from build123d import *

# Parameters (mm, degrees)
SKETCH1_R               = 4.60375
BOSS_EXTRUDE1_DEPTH     = 2.54
SKETCH2_R               = 3.175
BOSS_EXTRUDE2_DEPTH     = 45.72
SKETCH3_R               = 1.27
CUT_EXTRUDE1_DEPTH      = 5.60375
CUT_EXTRUDE1_DEPTH_BACK = 5.60375
FILLET1_R               = 0.635
CHAMFER1_SIZE           = 0.635
SKETCH4_W               = 16.845680721
SKETCH4_H               = 19.604839444
CUT_EXTRUDE2_DEPTH      = 5.60375
CUT_EXTRUDE2_DEPTH_BACK = 5.6037501


with BuildPart() as part:
    # Sketch1 → Boss-Extrude1 (new body)
    with BuildSketch(Plane(origin=(0, 0, 0), x_dir=(1, 0, 0), z_dir=(0, 1, 0))):
        Circle(SKETCH1_R)
    extrude(amount=BOSS_EXTRUDE1_DEPTH)

    # Sketch2 → Boss-Extrude2 (add)
    with BuildSketch(Plane(origin=(0, 2.54, 0), x_dir=(1, 0, 0), z_dir=(0, 1, 0))):
        Circle(SKETCH2_R)
    extrude(amount=BOSS_EXTRUDE2_DEPTH)

    # Sketch3 → Cut-Extrude1 (cut, two sides)
    with BuildSketch(Plane.XY) as cut_extrude1_sk:
        with Locations((0, 18.415)):
            Circle(SKETCH3_R)
        with Locations((0, 23.495)):
            Circle(SKETCH3_R)
        with Locations((0, 28.575)):
            Circle(SKETCH3_R)
        with Locations((0, 33.655)):
            Circle(SKETCH3_R)
        with Locations((0, 38.735)):
            Circle(SKETCH3_R)
        with Locations((0, 43.815)):
            Circle(SKETCH3_R)
    extrude(amount=CUT_EXTRUDE1_DEPTH, mode=Mode.SUBTRACT)
    extrude(cut_extrude1_sk.sketch, amount=-CUT_EXTRUDE1_DEPTH_BACK, mode=Mode.SUBTRACT)

    # Fillet1
    fillet1_edges = [part.edges().sort_by_distance(p)[0] for p in [
        (-4.60375, 2.54, 0),
    ]]
    fillet(fillet1_edges, radius=FILLET1_R)

    # Chamfer1
    chamfer1_edges = [part.edges().sort_by_distance(p)[0] for p in [
        (-4.60375, 0, 0),
    ]]
    chamfer(chamfer1_edges, length=CHAMFER1_SIZE)

    # Sketch4 → Cut-Extrude2 (cut, two sides)
    with BuildSketch(Plane(origin=(0, 0, 0), x_dir=(0, 0, -1), z_dir=(1, 0, 0))) as cut_extrude2_sk:
        with Locations((1.010740844, 42.122953468)):
            Rectangle(SKETCH4_W, SKETCH4_H)
    extrude(amount=CUT_EXTRUDE2_DEPTH, mode=Mode.SUBTRACT)
    extrude(cut_extrude2_sk.sketch, amount=-CUT_EXTRUDE2_DEPTH_BACK, mode=Mode.SUBTRACT)


solid = part.part
Verification items for the finished model (mm, model axes). A direction names the side the tool comes from. Coordinates: 2 decimals unless noted, no trailing zeros. Order: outer loops, then holes, each group sorted by start corner. A loop starts at its lowest first (then second) coordinate and runs counter-clockwise, first axis right, second up. Notation, with made-up numbers: (-12, 16.25) -> (17, 16.25) arc R38 cw to (17, 54.25) -> close; hole circle Ø9 at (89.5, 29). An arc over 180 degrees is marked (long way). Use CSV: the item, a comma, the result in double quotes. Start each with the question number.
Q1. Tool access check on faces 1 (the cylindrical face through (-0.275, 27.335, 0.044)), 2 (the cylindrical face through (1.5, 17.2, 2.8)). Record the directions out of +Z, -Z, +X, -X, +Y, -Y that give a thin tool (end or side, any length) a straight path to the whole face; none if there is none.
Q2. Section check C-C, the plane y = 6. Record the cut outline in (x, z) (3 decimals).
Q3. Section check B-B, the plane z = 0. Record the cut outline in (x, y) (3 decimals), and give its area (3 significant figures).
Q4. Depth check by flat-ended pin: P1, Ø1, axis at x = 1.5, y = 14, coming from the -Z side; P2, Ø3.5, axis at x = 0, y = 23.495, coming from the +Z side (3 decimals). Enter the tip coordinate at first touch or a pass-through.
Q5. Section check D-D, the plane z = 2.5. Give the number of separate pieces and of enclosed holes in the cut face, and give its area (3 significant figures).
Q6. Thickness scan on line 1 along Y through (x, z) = (0, 2) (3 decimals); line 2 along Y through (x, z) = (0.25, -0.5); line 3 along X through (y, z) = (14, 0) (3 decimals). Record the ranges inside material, lowest first.
Q7. Draft check along X on faces 3 (the cylindrical face through (-0.165, 19.674, 0.044)), 4 (the cylindrical face through (-3.653, 1.261, 2.801)), 5 (the flat face through (-2, 2.54, -3)). Enter one of: +X half, -X half, draft (parallel to the pull), parting line (faces both ways), or undercut.
Q8. Section check A-A, the plane x = 0. Record the cut outline in (y, z) (3 decimals), and give its area (3 significant figures).
Returned:
1,face 1,"+Z, -Z"
1,face 2,"+Y"
2,outline,"circle Ø6.35 at (0, 0)"
3,outline,"(-4.604, 0.635) -> (-3.969, 0) -> (3.969, 0) -> (4.604, 0.635) -> (4.604, 1.905) arc R0.635 ccw to (3.969, 2.54) -> (3.175, 2.54) -> (3.175, 32.321) -> (-3.175, 32.321) -> (-3.175, 2.54) -> (-3.969, 2.54) arc R0.635 ccw to (-4.604, 1.905) -> close; hole circle Ø2.54 at (0, 18.415); hole circle Ø2.54 at (0, 23.495); hole circle Ø2.54 at (0, 28.575)"
3,area,"197 mm^2"
4,P1,"stops at z = -3.01"
4,P2,"stops at z = 3.175"
5,separate pieces,"1"
5,enclosed holes,"3"
5,area,"120 mm^2"
6,line 1,"y = 0 to 17.145, 19.685 to 22.225, 24.765 to 27.305, 29.845 to 32.321"
6,line 2,"y = 0 to 17.17, 19.66 to 22.25, 24.74 to 27.33, 29.82 to 32.32"
6,line 3,"x = -3.175 to 3.175"
7,face 3,"undercut"
7,face 4,"parting line"
7,face 5,"draft"
8,outline,"(0, -3.969) -> (0.635, -4.604) -> (1.905, -4.604) arc R0.635 ccw to (2.54, -3.969) -> (2.54, -3.175) -> (17.145, -3.175) -> (17.145, 3.175) -> (2.54, 3.175) -> (2.54, 3.969) arc R0.635 ccw to (1.905, 4.604) -> (0.635, 4.604) -> (0, 3.969) -> close; (19.685, -3.175) -> (22.225, -3.175) -> (22.225, 3.175) -> (19.685, 3.175) -> close; (24.765, -3.175) -> (27.305, -3.175) -> (27.305, 3.175) -> (24.765, 3.175) -> close; (29.845, -3.175) -> (32.321, -3.175) -> (32.321, 3.175) -> (29.845, 3.175) -> close"
8,area,"164 mm^2"
